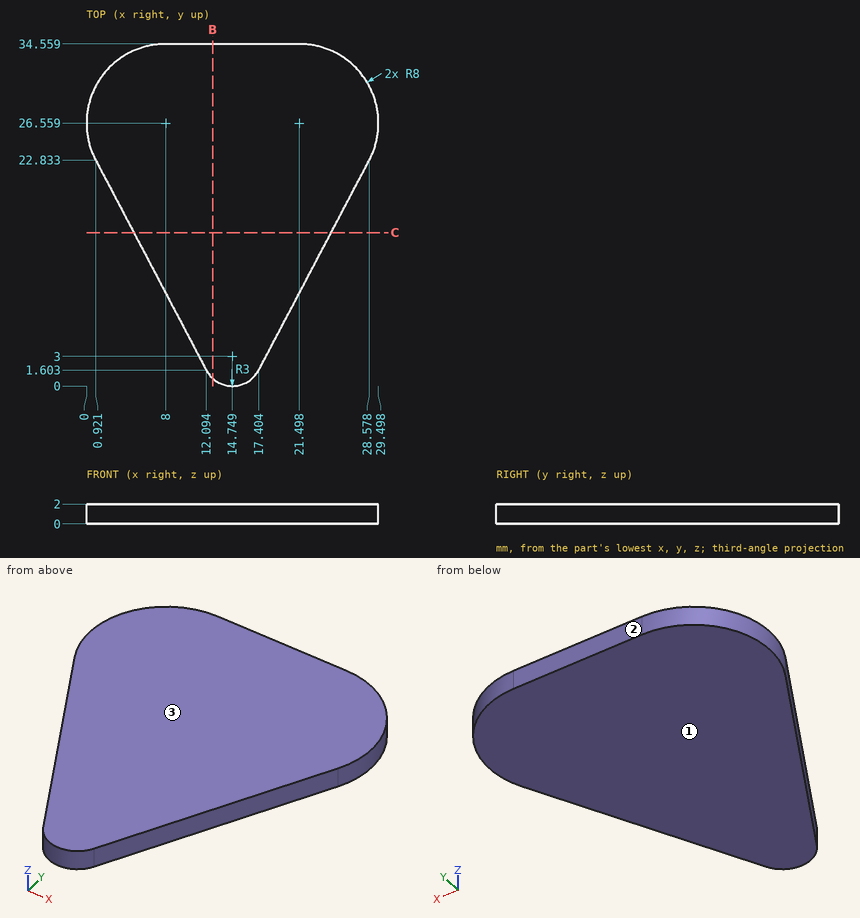
Input: dimensioned drawing with shaded views. Units: mm. Origin: part minimum x, y, z. Round coordinates to 2 decimals unless told otherwise and drop trailing zeros. Order: outer loops, then holes, each group sorted by start corner. A loop starts at its lowest first (then second) coordinate and runs counter-clockwise, first axis right, second up. Notation, with made-up numbers: (29.25, 68) -> (48.25, 68) arc R16 ccw to (48.25, 83) -> close; hole circle Ø6 at (-14, -27.75). An arc over 180 degrees is marked (long way). One line per item, written item: value. Start each with the question number.
Q1. Material intervals for probe 1 along Y at (x, z) = (5.5, 1.3) (1 decimal); probe 2 along X at (y, z) = (15, 0.65) (1 decimal); probe 3 along Y at (x, z) = (3.75, 1.1) (1 decimal), sorted ascending.
Q2. Section query C-C (y = 15.5). Return the cut outline in (x, z).
Q3. Section query B-B (x = 12.75). Return the cut outline in (y, z).
Q4. Draft query along Z for the marked faces 1, 2 and 3. Return one class per face: pulls with the +Z half, pulls with the -Z half, needs draft (parallel to the pull), parting line crosses it, or undercut.
Findings below:
1. probe 1: 14.1 to 34.2
1. probe 2: 5 to 24.5
1. probe 3: 17.5 to 33.3
2. outline: (4.78, 0) -> (24.72, 0) -> (24.72, 2) -> (4.78, 2) -> close
3. outline: (0.76, 0) -> (34.56, 0) -> (34.56, 2) -> (0.76, 2) -> close
4. face 1: pulls with the -Z half
4. face 2: needs draft
4. face 3: pulls with the +Z half
